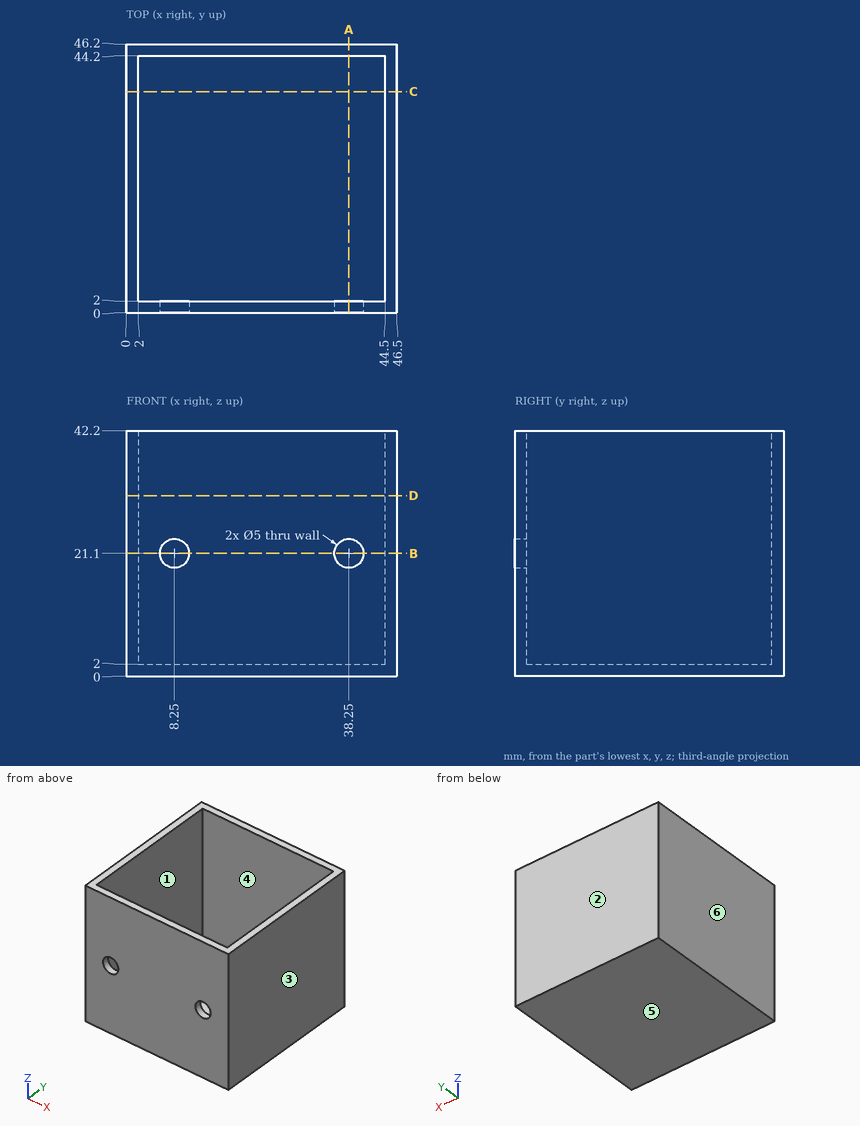
Print and shaded views of the part. All mm, measured from the part's lowest x, y and z. A direction names the side the tool comes from. Coordinates: 2 decimals unless noted, no trailing zeros. Order: outer loops, then holes, each group sorted by start corner. A loop starts at its lowest first (then second) coordinate and runs counter-clockwise, first axis right, second up.
(1) Probe L1, parallel to X at y = 0.65, z = 21.1; L2, parallel to Y at x = 44, z = 40; L3, parallel to X at y = 6, z = 9. List the from-to ranges inside material, lowest first.
Check sheet entries:
L1: x = 0 to 5.75, 10.75 to 35.75, 40.75 to 46.5
L2: y = 0 to 2, 44.2 to 46.2
L3: x = 0 to 2, 44.5 to 46.5
(2) Slice it at C-C, the plane y = 38. Write the cut outline in (x, z), and give its area (3 significant figures).
Check sheet entries:
outline: (0, 0) - (46.5, 0) - (46.5, 42.2) - (44.5, 42.2) - (44.5, 2) - (2, 2) - (2, 42.2) - (0, 42.2) - close
area: 254 mm2
(3) Slice it at D-D, the plane z = 31. Write the cut outline in (x, y), and give its area (3 significant figures).
Check sheet entries:
outline: (0, 0) - (46.5, 0) - (46.5, 46.2) - (0, 46.2) - close; hole (2, 2) - (44.5, 2) - (44.5, 44.2) - (2, 44.2) - close
area: 355 mm2
(4) Tool access for the marked faces 1 and 2: list every direction of +Z, -Z, +X, -X, +Y, -Y with a clear straight run to the whole face (end or side of a thin tool).
Check sheet entries:
face 1: +Z
face 2: +Z, -Z, +X, -X, +Y
(5) Pin check, flat tip, straight feed: pin 1 Ø4 at (x, y) = (32.5, 29) entering from +Z. Stop position of the tip, or through.
Check sheet entries:
pin 1: stops at z = 2
(6) Slice it at A-A, the plane x = 38.25. Write the cut outline in (y, z).
Check sheet entries:
outline: (0, 0) - (46.2, 0) - (46.2, 42.2) - (44.2, 42.2) - (44.2, 2) - (2, 2) - (2, 18.6) - (0, 18.6) - close; (0, 23.6) - (2, 23.6) - (2, 42.2) - (0, 42.2) - close
(7) Pull direction X, two halves, no side cores. Call the marked faces 3, 4, 5 and 6: pulls with the +X half, pulls with the -X half, needs draft (parallel to the pull), parting line crosses it, or undercut.
Check sheet entries:
face 3: pulls with the +X half
face 4: undercut
face 5: needs draft
face 6: pulls with the -X half
(8) Slice it at B-B, the plane z = 21.1. Write the cut outline in (x, y), and give its area (3 significant figures).
Check sheet entries:
outline: (0, 0) - (5.75, 0) - (5.75, 2) - (2, 2) - (2, 44.2) - (44.5, 44.2) - (44.5, 2) - (40.75, 2) - (40.75, 0) - (46.5, 0) - (46.5, 46.2) - (0, 46.2) - close; (10.75, 0) - (35.75, 0) - (35.75, 2) - (10.75, 2) - close
area: 335 mm2
